Here's how the part is built. I have some questions about the finished solid (model axes, mm). Round coordinates to 2 decimals unless told otherwise and drop trailing zeros. Order: outer loops, then holes, each group sorted by start corner. A loop starts at its lowest first (then second) coordinate and runs counter-clockwise, first axis right, second up. Notation, with made-up numbers: (8.25, 1) - (65.25, 1) arc R22 cw to (65.25, 35) - close; hole circle Ø5 at (-16, -30). An arc over 180 degrees is marked (long way). Answer as a JSON object with one key per item and string values.
```python
from build123d import *

# Parameters (mm, degrees)
BOSS_EXTRUDE1_DEPTH   = 5
M8_TAPPED_HOLE1_D     = 6.8
M8_TAPPED_HOLE1_DEPTH = 19.75
M8_TAPPED_HOLE1_TIP   = 2.042926105


with BuildPart() as part:
    # Sketch1 → Boss-Extrude1 (new body)
    with BuildSketch(Plane.XY):
        Polygon((9.913260994, -5.921198341), (10.084538681, 5.624536685), (0.171277687, 11.545735026), (-9.913260994, 5.921198341), (-10.084538681, -5.624536685), (-0.171277687, -11.545735026), align=None)
    extrude(amount=BOSS_EXTRUDE1_DEPTH)

    # M8 Tapped Hole1
    with Locations(Plane.XY.offset(5)):
        with Locations((0, 0)):
            Hole(M8_TAPPED_HOLE1_D / 2, depth=M8_TAPPED_HOLE1_DEPTH)
            with Locations((0, 0, -(M8_TAPPED_HOLE1_DEPTH + M8_TAPPED_HOLE1_TIP / 2))):  # 118° drill point
                Cone(0, M8_TAPPED_HOLE1_D / 2, M8_TAPPED_HOLE1_TIP, mode=Mode.SUBTRACT)


solid = part.part
```
1. Imagine slicing it at C-C (x = 6.5). List the corners of the cut face in (y, z) for me, plus the area to 3 significant figures.
Responses:
{"outline": "(-7.82, 0) - (7.77, 0) - (7.77, 5) - (-7.82, 5) - close", "area": "78.0 mm2"}
2. For P1, Ø1, axis at x = -3, z = 2.5, coming from the -Y side; P2, Ø3, axis at y = 7.5, z = 3.5, coming from the +X side; P3, Ø1, axis at y = -2, z = 0.5, coming from the +X side, each with a flat end and sliding along its axis, tell me the tip position at first contact or that it passes through.
Responses:
{"P1": "y = -10.15", "P2": "x = 9.46", "P3": "x = 9.98"}
3. Imagine slicing it at B-B (y = 0). List the corners of the cut face in (x, z) for me.
Responses:
{"outline": "(-10, 0) - (-3.4, 0) - (-3.4, 5) - (-10, 5) - close; (3.4, 0) - (10, 0) - (10, 5) - (3.4, 5) - close"}
4. If I drill on L1, parallel to Y at x = -1.5, z = 0.8; L2, parallel to Y at x = 0, z = 2.45; L3, parallel to X at y = 3, z = 4.8, over which ranges is the centre line in solid material (lowest first)? Write a range as [from, to].
Responses:
{"L1": "[-10.75, -3.05], [3.05, 10.61]", "L2": "[-11.45, -3.4], [3.4, 11.45]", "L3": "[-9.96, -1.6], [1.6, 10.05]"}
5. Thinking about a two-plate mould opening in Y: for faces 1 (the face through (-2, 3, 0)), 2 (the face through (0.74, -3.32, 2.46)), 3 (the face through (-4.8, 8.773, 2.465)), 4 (the face through (-5.2, -8.54, 2.46)), which applies, pulls with the +Y half, pulls with the -Y half, needs draft (parallel to the pull), parting line crosses it, or undercut?
Responses:
{"face 1": "needs draft", "face 2": "undercut", "face 3": "pulls with the +Y half", "face 4": "pulls with the -Y half"}
6. Imagine slicing it at A-A (z = 0.7). List the corners of the cut face in (x, y) for me, plus the area to 3 significant figures.
Responses:
{"outline": "(-10.08, -5.62) - (-0.17, -11.55) - (9.91, -5.92) - (10.08, 5.62) - (0.17, 11.55) - (-9.91, 5.92) - close; hole circle Ø6.8 at (0, 0)", "area": "310 mm2"}
7. Imagine slicing it at D-D (y = -3). List the corners of the cut face in (x, z) for me, plus the area to 3 significant figures.
Responses:
{"outline": "(-10.05, 0) - (-1.6, 0) - (-1.6, 5) - (-10.05, 5) - close; (1.6, 0) - (9.96, 0) - (9.96, 5) - (1.6, 5) - close", "area": "84.0 mm2"}
